from build123d import *

# Parameters (mm, degrees)
SKETCH2_W           = 6.604
SKETCH2_H           = 12.7
SKETCH2_W_2         = 2.54
SKETCH2_H_2         = 14.47
BOSS_EXTRUDE1_DEPTH = 12.7
SKETCH3_R           = 1.75
CUT_EXTRUDE1_DEPTH  = 32.27817965
BOSS_EXTRUDE4_START = -18.57818
SKETCH3_3_R         = 1.6
BOSS_EXTRUDE4_DEPTH = 12.7
CUT_EXTRUDE12_DEPTH = 13.70000035
CUT_EXTRUDE14_DEPTH = 3.048
SKETCH37_W          = 1.6
SKETCH37_H          = 28.71
CUT_EXTRUDE17_DEPTH = 3.175
SKETCH38_W          = 1.677757264
SKETCH38_H          = 8.39
BOSS_EXTRUDE7_DEPTH = 1.5875


with BuildPart() as part:
    # Sketch2 → Boss-Extrude1 (new body)
    with BuildSketch(Plane(origin=(0, 0, 0), x_dir=(1, 0, 0), z_dir=(0, 1, 0))):
        Polygon((-28.23017965, 12.02419618), (-31.27817965, 12.02419618), (-31.27817965, -3.98580382), (-28.73817965, -3.98580382), (-21.11817965, -3.98580382), (-18.57817965, -3.98580382), (-18.57817965, 12.02419618), (-21.62617965, 12.02419618), align=None)
        with Locations((-24.92817965, 18.37419618)):
            Rectangle(SKETCH2_W, SKETCH2_H)
        with Locations((-19.84817965, -11.22080382)):
            Rectangle(SKETCH2_W_2, SKETCH2_H_2)
        with Locations((-30.00817965, -11.22080382)):
            Rectangle(SKETCH2_W_2, SKETCH2_H_2)
    extrude(amount=BOSS_EXTRUDE1_DEPTH)

    # Sketch3 → Cut-Extrude1 (cut, through all)
    with BuildSketch(Plane(origin=(0, 0, 0), x_dir=(0, 0, -1), z_dir=(1, 0, 0))):
        with Locations((18.72419618, 6.35)):
            Circle(SKETCH3_R)
    extrude(amount=-CUT_EXTRUDE1_DEPTH, mode=Mode.SUBTRACT)

    # Sketch3<3> → Boss-Extrude4 (add, through all)
    with BuildSketch(Plane(origin=(0, 0, 0), x_dir=(0, 0, -1), z_dir=(1, 0, 0)).offset(BOSS_EXTRUDE4_START)):
        with Locations((-13.37580382, 6.35)):
            Circle(SKETCH3_3_R)
    extrude(amount=-BOSS_EXTRUDE4_DEPTH)

    # Sketch29 → Cut-Extrude12 (cut, through all)
    with BuildSketch(Plane(origin=(-18.57817965, 0, 0), x_dir=(0, 0, -1), z_dir=(1, 0, 0))):
        Polygon((-18.45580382, 6.35), (-10.83580382, 0), (-18.45580382, 0), align=None)
    extrude(amount=-CUT_EXTRUDE12_DEPTH, mode=Mode.SUBTRACT)

    # Sketch31 → Cut-Extrude14 (cut)
    with BuildSketch(Plane(origin=(-18.57817965, 0, 0), x_dir=(0, 0, -1), z_dir=(1, 0, 0))):
        Polygon((12.02419618, 8.039800124), (4.40419618, 0), (12.02419618, 0), align=None)
    extrude(amount=-CUT_EXTRUDE14_DEPTH, mode=Mode.SUBTRACT)

    # Sketch37 → Cut-Extrude17 (cut)
    with BuildSketch(Plane.XZ):
        with Locations((-24.92817965, -10.36919618)):
            Rectangle(SKETCH37_W, SKETCH37_H)
    extrude(amount=-CUT_EXTRUDE17_DEPTH, mode=Mode.SUBTRACT)

    # Sketch38 → Boss-Extrude7 (add)
    with BuildSketch(Plane.XZ):
        with Locations((-24.889301018, -0.20919618)):
            Rectangle(SKETCH38_W, SKETCH38_H)
    extrude(amount=-BOSS_EXTRUDE7_DEPTH)


solid = part.part
CAD build for the part. Positions are in the model's coordinates, mm. A direction names the side the tool comes from. Round coordinates to 2 decimals unless told otherwise and drop trailing zeros. Order: outer loops, then holes, each group sorted by start corner. A loop starts at its lowest first (then second) coordinate and runs counter-clockwise, first axis right, second up. Notation, with made-up numbers: (73, -7.5) - (85, -7.5) arc R16 cw to (85, 5.5) - close; hole circle Ø7 at (-28.5, -35.5). An arc over 180 degrees is marked (long way). Return JSON: item names as keys, results as strings.
(1) Wall check: probe 1 along X at (y, z) = (2, -5.5); probe 2 along X at (y, z) = (11.5, 7.5); probe 3 along X at (y, z) = (8.25, -22.5). Give the ranges that are in metal, low to high. Write a range as from..to.
Answer key:
{"probe 1": "x = -31.28..-25.73, -24.13..-18.58", "probe 2": "x = -31.28..-28.74, -21.12..-18.58", "probe 3": "x = -28.23..-21.63"}
(2) Cut at B-B (y = 12.25). Give the cut face in (x, z).
Answer key:
{"outline": "(-31.28, -12.02) - (-28.23, -12.02) - (-28.23, -24.72) - (-21.63, -24.72) - (-21.63, -12.02) - (-18.58, -12.02) - (-18.58, 18.46) - (-21.12, 18.46) - (-21.12, 3.99) - (-28.74, 3.99) - (-28.74, 18.46) - (-31.28, 18.46) - close"}
(3) Cut at C-C (z = -13.5). Give the cut face in (x, y) (3 decimals), then the cut area to 3 significant figures.
Answer key:
{"outline": "(-28.23, 0) - (-25.728, 0) - (-25.728, 3.175) - (-24.128, 3.175) - (-24.128, 0) - (-21.626, 0) - (-21.626, 12.7) - (-28.23, 12.7) - close", "area": "78.8 mm^2"}
(4) Cut at D-D (z = -8). Give the cut face in (x, y) (3 decimals).
Answer key:
{"outline": "(-31.278, 0) - (-25.728, 0) - (-25.728, 3.175) - (-24.128, 3.175) - (-24.128, 0) - (-21.626, 0) - (-21.626, 3.794) - (-18.578, 3.794) - (-18.578, 12.7) - (-31.278, 12.7) - close"}
(5) Pin check, flat tips, straight feed: pin 1 Ø1.5 at (x, y) = (-20, 10) entering from -Z; pin 2 Ø4 at (y, z) = (7.5, -18) entering from +X; pin 3 Ø1.5 at (y, z) = (7, -16) entering from -X. Stop position of each tip, or through.
Answer key:
{"pin 1": "stops at z = -12.02", "pin 2": "stops at x = -21.63", "pin 3": "stops at x = -28.23"}
(6) Tool access for faces 4 (the face through (-25, 1.588, 0)), 5 (the face through (-24.128, 2, -14)), 6 (the face through (-20, 10, -12.024)), 7 (the face through (-24.87, 7.7, 12.52)), 8 (the face through (-20.08, 4.08, -8.27)): list every direction of +Z, -Z, +X, -X, +Y, -Y with a clear straight run to the whole face (end or side of a thin tool).
Answer key:
{"face 4": "+Z, -Z", "face 5": "-Z", "face 6": "-Z, +X, +Y, -Y", "face 7": "none", "face 8": "-Z, +X, -Y"}
(7) Cut at A-A (x = -26.25). Give the cut face in (y, z), then the cut area to 3 significant figures.
Answer key:
{"outline": "(0, -24.72) - (12.7, -24.72) - (12.7, 3.99) - (0, 3.99) - close; circle Ø3.2 at (6.35, 13.38); hole circle Ø3.5 at (6.35, -18.72)", "area": "363 mm^2"}
(8) Pull direction X, two halves, no side cores. Call faces 1 (the face through (-25, 3.175, -10)), 2 (the face through (-24.88, 6.88, -20.39)), 3 (the face through (-28.23, 5, -17)): +X half, -X half, draft (parallel to the pull), parting line (faces both ways), or undercut.
Answer key:
{"face 1": "undercut", "face 2": "draft", "face 3": "-X half"}
